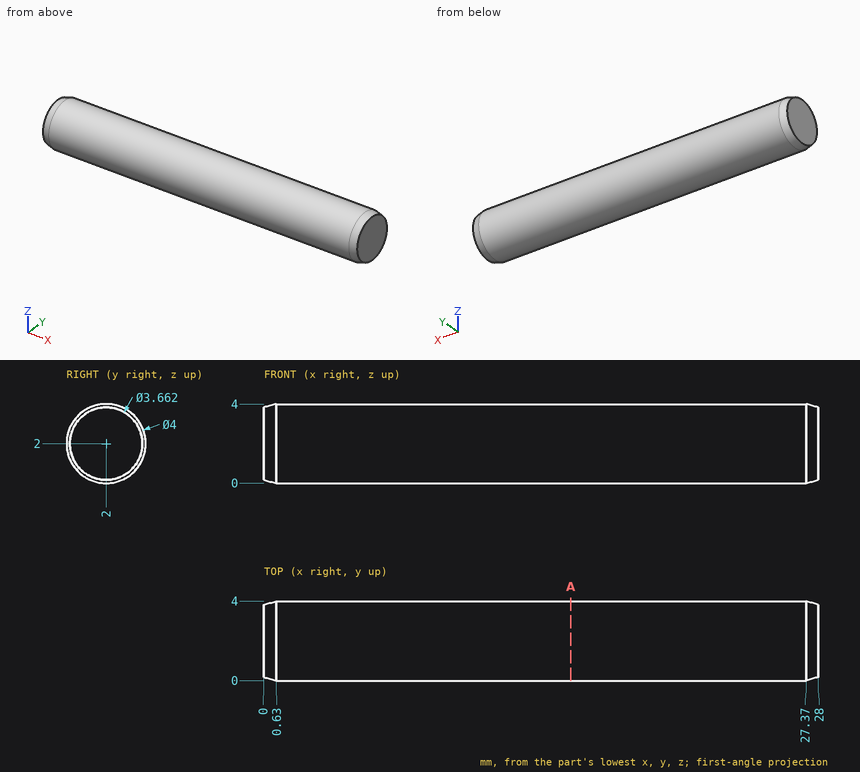
Geometry: see drawing. Coordinates: mm, zero at the bounding-box minimum. Coordinates: 2 decimals unless noted, no trailing zeros. Loops run counter-clockwise (first coordinate to the right, second up) from the corner with the lowest first, then second, coordinate; pieces in that order, holes last.
Q1. Contact query for flat-ended pins moving along their axis: pin 1 (1 mm diameter, centred on x = 18, z = 2.5, fed in from +Y); pin 2 (2 mm diameter, centred on x = 4.5, z = 3.5, fed in from -Y). Output: stop coordinate, or through.
Q2. Cut plane A-A (x = 15.5). Output: boundary loops of the cut face in (y, z).
Q3. Material intervals for line 1 (Z direction, x = 13.5, y = 2.8); line 2 (Y direction, x = 11.75, z = 2.15) (1 decimal), sorted ascending.
Working result:
1. pin 1: stops at y = 4
1. pin 2: stops at y = 0.06
2. outline: circle Ø4 at (2, 2)
3. line 1: z = 0.17 to 3.83
3. line 2: y = 0 to 4
